Source: three-view drawing plus pictorial views. Frame: mm from the lowest corner of the part. A direction names the side the tool comes from. Round coordinates to 2 decimals unless told otherwise and drop trailing zeros. Order: outer loops, then holes, each group sorted by start corner. A loop starts at its lowest first (then second) coordinate and runs counter-clockwise, first axis right, second up. Notation, with made-up numbers: (47.5, -38) - (59.5, -38) arc R14 ccw to (59.5, -20) - close; hole circle Ø11 at (57, 13). An arc over 180 degrees is marked (long way). Use one line per item in the form item = value. Start each with the question number.
Q1. Cut plane C-C, the plane z = 26.5. Return the cut outline in (x, y).
Q2. Draft query along X for the marked faces 1, 2 and 3. Return one class per face: released by +X, released by -X, zero draft, split by the parting line, or undercut.
Q3. Ray query, line 1 (Z direction, x = 20.1, y = 6); line 2 (Z direction, x = 20.1, y = 2.5); line 3 (X direction, y = 8, z = 30). Return the intervals inside material, ascending. Write a range as [from, to].
Q4. Cut plane D-D, the plane y = 1. Return the cut outline in (x, z).
Q5. Cut plane B-B, the plane z = 20.1. Return the cut outline in (x, y), and give its area (3 significant figures).
Q6. Cut plane A-A, the plane x = 20.1. Return the cut outline in (y, z), and give its area (3 significant figures).
Q7. Set-up query: the marked faces 4 and 5. Return all of +Z, -Z, +X, -X, +Y, -Y with unobstructed straight access to the full face (end or side cutting, diameter ignored); none if empty.
Q8. Pin query (flat end, axial travel): pin 1 Ø5 at (y, z) = (8, 31.5) entering from -X; pin 2 Ø6 at (x, y) = (34, 8.5) entering from +Z; pin 3 Ø4 at (x, z) = (20.1, 4.5) entering from -Y; pin 4 Ø4 at (x, y) = (24.5, 2.5) entering from -Z. Return the tip coordinate at first contact, or that it passes through.
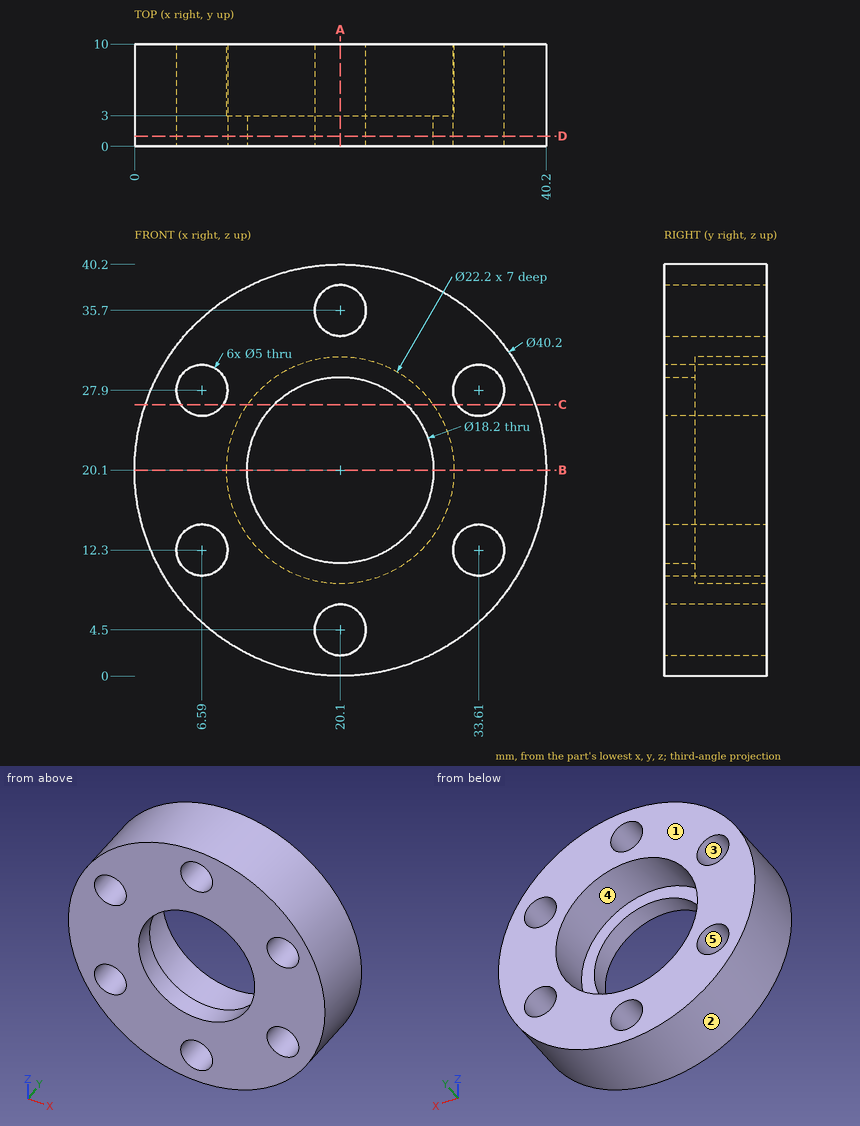
Completed:
q1.outline = (1.05, 0) - (4.52, 0) - (4.52, 10) - (1.05, 10) - close; (8.66, 0) - (13.63, 0) - (13.63, 3) - (11.03, 3) - (11.03, 10) - (8.66, 10) - close; (26.57, 0) - (31.54, 0) - (31.54, 10) - (29.17, 10) - (29.17, 3) - (26.57, 3) - close; (35.68, 0) - (39.15, 0) - (39.15, 10) - (35.68, 10) - close
q2.face_1 = zero draft
q2.face_2 = split by the parting line
q2.face_3 = undercut
q3.line_1 = [0, 2], [7, 9], [31.2, 33.2], [38.2, 40.2]
q3.line_2 = [0, 2], [7, 11], [29.2, 33.2], [38.2, 40.2]
q3.line_3 = [2.61, 5.23], [7.95, 15.08], [25.12, 32.25], [34.97, 37.59]
q4.outline = circle Ø40.2 at (20.1, 20.1); hole circle Ø5 at (6.59, 12.3); hole circle Ø5 at (6.59, 27.9); hole circle Ø18.2 at (20.1, 20.1); hole circle Ø5 at (20.1, 4.5); hole circle Ø5 at (20.1, 35.7); hole circle Ø5 at (33.61, 12.3); hole circle Ø5 at (33.61, 27.9)
q5.outline = (0, 0) - (11, 0) - (11, 3) - (9, 3) - (9, 10) - (0, 10) - close; (29.2, 0) - (40.2, 0) - (40.2, 10) - (31.2, 10) - (31.2, 3) - (29.2, 3) - close
q5.area = 192 mm2
q6.outline = (0, 0) - (10, 0) - (10, 2) - (0, 2) - close; (0, 7) - (10, 7) - (10, 9) - (3, 9) - (3, 11) - (0, 11) - close; (0, 29.2) - (3, 29.2) - (3, 31.2) - (10, 31.2) - (10, 33.2) - (0, 33.2) - close; (0, 38.2) - (10, 38.2) - (10, 40.2) - (0, 40.2) - close
q6.area = 92.0 mm2
q7.face_4 = +Y
q7.face_5 = +Y, -Y
q8.pin_1 = 2.08
q8.pin_2 = 36.99
q8.pin_3 = through
q8.pin_4 = 0.14
